CAD build for the part. Positions are in the model's coordinates, mm. A direction names the side the tool comes from. Coordinates: 2 decimals unless noted, no trailing zeros. Write each loop counter-clockwise with the first axis right and the second up, starting at its lowest first coordinate (ties: lowest second). Pieces come first, ordered by that corner, then holes. Notation, with made-up numbers: M 87,71.25 L 139,71.25 A26 cw 139,93.25 Z; hole C 53.25,60.25 d11. An arc over 180 degrees is marked long. Answer as CSV lines item,"result". Start each with the question number.
```python
from build123d import *

# Parameters (mm, degrees)
SKETCH1_W             = 94.85
SKETCH1_H             = 94.85
SKETCH1_W_2           = 88.85
SKETCH1_H_2           = 88.85
BOSS_EXTRUDE1_DEPTH   = 5
SKETCH1_W_3           = 81.5
SKETCH1_H_3           = 81.5
BOSS_EXTRUDE1_2_DEPTH = 5
SKETCH2_W             = 94.85
SKETCH2_H             = 94.85
BOSS_EXTRUDE2_DEPTH   = 2


with BuildPart() as part:
    # Sketch1 → Boss-Extrude1 (new body)
    with BuildSketch(Plane(origin=(0, 0, 0), x_dir=(1, 0, 0), z_dir=(0, 1, 0))):
        with Locations((40.75, 40.75)):
            Rectangle(SKETCH1_W, SKETCH1_H)
        with Locations((40.75, 40.75)):
            Rectangle(SKETCH1_W_2, SKETCH1_H_2, mode=Mode.SUBTRACT)
    extrude(amount=BOSS_EXTRUDE1_DEPTH)



with BuildPart() as body_2:
    # Sketch1 → Boss-Extrude1 2 (new body)
    with BuildSketch(Plane(origin=(0, 0, 0), x_dir=(1, 0, 0), z_dir=(0, 1, 0))):
        with Locations((40.75, 40.75)):
            Rectangle(SKETCH1_W_3, SKETCH1_H_3)
    extrude(amount=BOSS_EXTRUDE1_2_DEPTH)


with BuildPart() as part_1:
    add(part.part)

    add(body_2.part)  # Boss-Extrude2 merges body 2
    # Sketch2 → Boss-Extrude2 (add)
    with BuildSketch(Plane.XZ):
        with Locations((40.75, -40.75)):
            Rectangle(SKETCH2_W, SKETCH2_H)
    extrude(amount=BOSS_EXTRUDE2_DEPTH)


solid = part_1.part
```
1) Band-saw the part on B-B, the plane z = -41.5. List the corners of the cut face in (x, y) (3 decimals), plus the area to 3 significant figures.
2) Probe L1, parallel to Z at x = 63.5, y = 4.25 (3 decimals); L2, parallel to X at y = 3, z = -79 (3 decimals); L3, parallel to X at y = 4.25, z = 1 (3 decimals). List the from-to ranges inside material, lowest first. Write a range as [from, to].
3) Band-saw the part on A-A, the plane y = 3.5. List the corners of the cut face in (x, z) (3 decimals).
4) Tool access for faces 1 (the flat face through (-3.675, 2, -40)), 2 (the flat face through (-6.675, 2, -41)): list every direction of +Z, -Z, +X, -X, +Y, -Y with a clear straight run to the whole face (end or side of a thin tool).
5) Two-plate mould, pull along Z, no slides. Class faces 3 (the flat face through (40, 2, -85.175)), 4 (the flat face through (40, 2, -81.5)), 5 (the flat face through (40, 2, -88.175)), 6 (the flat face through (40, 5, -41)): pulls with the +Z half, pulls with the -Z half, needs draft (parallel to the pull), parting line crosses it, or undercut.
6) Band-saw the part on C-C, the plane x = 41.5. List the corners of the cut face in (y, z) (3 decimals), plus the area to 3 significant figures.
Result sheet:
1,outline,"M -6.675,-2 L 88.175,-2 L 88.175,5 L 85.175,5 L 85.175,0 L 81.5,0 L 81.5,5 L 0,5 L 0,0 L -3.675,0 L -3.675,5 L -6.675,5 Z"
1,area,"627 mm²"
2,L1,"z = [-88.175, -85.175], [-81.5, 0], [3.675, 6.675]"
2,L2,"x = [-6.675, -3.675], [0, 81.5], [85.175, 88.175]"
2,L3,"x = [-6.675, -3.675], [85.175, 88.175]"
3,outline,"M -6.675,-88.175 L 88.175,-88.175 L 88.175,6.675 L -6.675,6.675 Z; M 0,-81.5 L 81.5,-81.5 L 81.5,0 L 0,0 Z; hole M -3.675,-85.175 L 85.175,-85.175 L 85.175,3.675 L -3.675,3.675 Z"
4,face 1,"+Y"
4,face 2,"+Z, -Z, -X, +Y, -Y"
5,face 3,"undercut"
5,face 4,"undercut"
5,face 5,"pulls with the -Z half"
5,face 6,"needs draft"
6,outline,"M -2,-88.175 L 5,-88.175 L 5,-85.175 L 0,-85.175 L 0,-81.5 L 5,-81.5 L 5,0 L 0,0 L 0,3.675 L 5,3.675 L 5,6.675 L -2,6.675 Z"
6,area,"627 mm²"
